from build123d import *

# Parameters (mm, degrees)
SKETCH1_W           = 130
SKETCH1_H           = 55
SKETCH1_R           = 1.6
SKETCH1_R_2         = 8
BOSS_EXTRUDE4_DEPTH = 3.5
FILLET4_R           = 10


with BuildPart() as part:
    # Sketch1 → Boss-Extrude4 (new body)
    with BuildSketch(Plane(origin=(0, 0, 0), x_dir=(1, 0, 0), z_dir=(0, 1, 0))):
        with Locations((65, -27.5)):
            Rectangle(SKETCH1_W, SKETCH1_H)
        with Locations((9, -12.5)):
            Circle(SKETCH1_R, mode=Mode.SUBTRACT)
        with Locations((9, -42.5)):
            Circle(SKETCH1_R, mode=Mode.SUBTRACT)
        with Locations((121, -42.5)):
            Circle(SKETCH1_R, mode=Mode.SUBTRACT)
        with Locations((121, -12.5)):
            Circle(SKETCH1_R, mode=Mode.SUBTRACT)
        with Locations((15, -27.5)):
            Circle(SKETCH1_R_2, mode=Mode.SUBTRACT)
        with Locations((115, -27.5)):
            Circle(SKETCH1_R_2, mode=Mode.SUBTRACT)
        with Locations((65, -12.425)):
            Circle(SKETCH1_R, mode=Mode.SUBTRACT)
        with Locations((65, -42.575)):
            Circle(SKETCH1_R, mode=Mode.SUBTRACT)
        with Locations((75, -12.425)):
            Circle(SKETCH1_R, mode=Mode.SUBTRACT)
        with Locations((75, -42.575)):
            Circle(SKETCH1_R, mode=Mode.SUBTRACT)
        with Locations((85, -12.425)):
            Circle(SKETCH1_R, mode=Mode.SUBTRACT)
        with Locations((85, -42.575)):
            Circle(SKETCH1_R, mode=Mode.SUBTRACT)
        with Locations((95, -12.425)):
            Circle(SKETCH1_R, mode=Mode.SUBTRACT)
        with Locations((95, -42.575)):
            Circle(SKETCH1_R, mode=Mode.SUBTRACT)
        with Locations((105, -12.425)):
            Circle(SKETCH1_R, mode=Mode.SUBTRACT)
        with Locations((105, -42.575)):
            Circle(SKETCH1_R, mode=Mode.SUBTRACT)
        with Locations((55, -12.425)):
            Circle(SKETCH1_R, mode=Mode.SUBTRACT)
        with Locations((55, -42.575)):
            Circle(SKETCH1_R, mode=Mode.SUBTRACT)
        with Locations((45, -12.425)):
            Circle(SKETCH1_R, mode=Mode.SUBTRACT)
        with Locations((45, -42.575)):
            Circle(SKETCH1_R, mode=Mode.SUBTRACT)
        with Locations((35, -12.425)):
            Circle(SKETCH1_R, mode=Mode.SUBTRACT)
        with Locations((35, -42.575)):
            Circle(SKETCH1_R, mode=Mode.SUBTRACT)
        with Locations((25, -12.425)):
            Circle(SKETCH1_R, mode=Mode.SUBTRACT)
        with Locations((25, -42.575)):
            Circle(SKETCH1_R, mode=Mode.SUBTRACT)
        with Locations((65, -27.5)):
            Circle(SKETCH1_R, mode=Mode.SUBTRACT)
        with Locations((75, -27.5)):
            Circle(SKETCH1_R, mode=Mode.SUBTRACT)
        with Locations((85, -27.5)):
            Circle(SKETCH1_R, mode=Mode.SUBTRACT)
        with Locations((95, -27.5)):
            Circle(SKETCH1_R, mode=Mode.SUBTRACT)
        with Locations((55, -27.5)):
            Circle(SKETCH1_R, mode=Mode.SUBTRACT)
        with Locations((45, -27.5)):
            Circle(SKETCH1_R, mode=Mode.SUBTRACT)
        with Locations((35, -27.5)):
            Circle(SKETCH1_R, mode=Mode.SUBTRACT)
        with Locations((28, -27.5)):
            Circle(SKETCH1_R, mode=Mode.SUBTRACT)
        with Locations((102, -27.5)):
            Circle(SKETCH1_R, mode=Mode.SUBTRACT)
    extrude(amount=BOSS_EXTRUDE4_DEPTH)

    # Fillet4
    fillet4_edges = [part.edges().sort_by_distance(p)[0] for p in [
        (0, 1.75, 0),
        (130, 1.75, 0),
        (130, 1.75, 55),
        (0, 1.75, 55),
    ]]
    fillet(fillet4_edges, radius=FILLET4_R)


solid = part.part
Design review of the part built by this model. Coordinates are the model's own, in mm. Give positions to 0.01 mm unless a question says otherwise; leave off trailing zeros. Loops run counter-clockwise (first coordinate to the right, second up) from the corner with the lowest first, then second, coordinate; pieces in that order, holes last. Notation, with made-up numbers: M 29.25,48 L 56.25,48 A32 ccw 56.25,87 Z; hole C -21.75,75 d11. An arc over 180 degrees is marked long. Answer as a JSON object with one key per item and string values.
Item 1: Mouldability with a two-part tool opening along X and no side actions: class faces 1 (the face through (93.4, 1.7, 12.4)), 2 (the face through (64, 3.5, 21)), 3 (the face through (126.99, 1.77, 2.85)), 4 (the face through (76.526, 1.726, 11.944)) as pulls with the +X half, pulls with the -X half, needs draft (parallel to the pull), parting line crosses it, or undercut.
Output values:
{"face 1": "undercut", "face 2": "needs draft", "face 3": "pulls with the +X half", "face 4": "undercut"}
Item 2: We need section D-D (z = 27.5). Count the separate pieces of the cut face and the enclosed holes in it, and give its area (3 significant figures).
Output values:
{"separate pieces": "12", "enclosed holes": "0", "area": "242 mm2"}
Item 3: We need section B-B (x = 15). State the section outline as (y, z) points, and give its area (4 significant figures).
Output values:
{"outline": "M 0,0 L 3.5,0 L 3.5,19.5 L 0,19.5 Z; M 0,35.5 L 3.5,35.5 L 3.5,55 L 0,55 Z", "area": "136.5 mm2"}
Item 4: We need section A-A (x = 85). State the section outline as (y, z) points (3 decimals), and give its area (3 significant figures).
Output values:
{"outline": "M 0,0 L 3.5,0 L 3.5,10.825 L 0,10.825 Z; M 0,14.025 L 3.5,14.025 L 3.5,25.9 L 0,25.9 Z; M 0,29.1 L 3.5,29.1 L 3.5,40.975 L 0,40.975 Z; M 0,44.175 L 3.5,44.175 L 3.5,55 L 0,55 Z", "area": "159 mm2"}
Item 5: We need section C-C (z = 33). State the section outline as (x, y) points.
Output values:
{"outline": "M 0,0 L 9.19,0 L 9.19,3.5 L 0,3.5 Z; M 20.81,0 L 109.19,0 L 109.19,3.5 L 20.81,3.5 Z; M 120.81,0 L 130,0 L 130,3.5 L 120.81,3.5 Z"}
Item 6: Wall thickness on line 1 along Z through (x, y) = (95, 1.65) (3 decimals); line 2 along Z through (x, y) = (9, 2.7); line 3 along X through (y, z) = (2.5, 34.5): over which ranges is each line inside the solid? List them lowest first.
Output values:
{"line 1": "z = 0 to 10.825, 14.025 to 25.9, 29.1 to 40.975, 44.175 to 55", "line 2": "z = 0.05 to 10.9, 14.1 to 22.21, 32.79 to 40.9, 44.1 to 54.95", "line 3": "x = 0 to 11.13, 18.87 to 111.13, 118.87 to 130"}
Item 7: For P1, Ø3, axis at x = 9, z = 12.5, coming from the -Y side; P2, Ø2, axis at y = 0.5, z = 48.5, coming from the -X side, all flat-tipped, find the tip position at first contact; note any pin that passes through.
Output values:
{"P1": "passes through", "P2": "stops at x = 0.32"}
